```python
from build123d import *

# Parameters (mm, degrees)
BOSS_EXTRUDE1_START     = -1.5
BOSS_EXTRUDE1_DEPTH     = 1.8
SKETCH8_R               = 3
SKETCH8_R_2             = 2.5
BOSS_EXTRUDE2_DEPTH     = 1.2
CUT_EXTRUDE1_DEPTH      = 9.631338251
CUT_EXTRUDE1_DEPTH_BACK = 9.631338251
SKETCH9_R               = 2.5
FILLET1_R               = 0.254
SWEEP1_PITCH            = 0.8
SPLIT1_START            = -2.7460001
SPLIT1_OUTLINE_W        = 9
SPLIT1_OUTLINE_H        = 2.5
SPLIT1_DEPTH            = 5.4920002


with BuildPart() as part:
    # Sketch7 → Boss-Extrude1 (new body)
    with BuildSketch(Plane.XY.offset(BOSS_EXTRUDE1_START)):
        with BuildLine():
            Line((-6.42820323, 4), (6.42820323, 4))
            ThreePointArc((6.42820323, 4), (7.5, 0), (6.42820323, -4))
            Line((6.42820323, -4), (-6.42820323, -4))
            ThreePointArc((-6.42820323, -4), (-7.5, 0), (-6.42820323, 4))
        make_face()
    extrude(amount=BOSS_EXTRUDE1_DEPTH)

    # Sketch8 → Boss-Extrude2 (add)
    with BuildSketch(Plane.XY.offset(0.3)):
        with Locations((1.5, 0)):
            Circle(SKETCH8_R)
        with Locations((1.5, 0)):
            Circle(SKETCH8_R_2, mode=Mode.SUBTRACT)
    extrude(amount=BOSS_EXTRUDE2_DEPTH)

    # Sketch9 → Cut-Extrude1 (cut, two sides: drawn at the far end of the back side and taken through both)
    with BuildSketch(Plane.XY.offset(-CUT_EXTRUDE1_DEPTH_BACK)):
        with Locations((1.5, 0)):
            Circle(SKETCH9_R)
    extrude(amount=CUT_EXTRUDE1_DEPTH + CUT_EXTRUDE1_DEPTH_BACK, mode=Mode.SUBTRACT)

    # Fillet1
    fillet1_edges = [part.edges().sort_by_distance(p)[0] for p in [
        (-1.5, 0, 1.5),
    ]]
    fillet(fillet1_edges, radius=FILLET1_R)

    # Sweep1: arcs per turn and ends read off the stored shape
    # Sweep1: the profile of Sketch3 screwed along a right-hand helix through 4.75 turns, 8 arcs to a turn; built about Z, then put on its axis
    sweep1_z = Axis((0, 0, 0), (0, 0, 1))
    sweep1_corners = [(2.54330127, 0, 0.025), (2.54330127, 0, -0.725), (1.980384758, 0, -0.4), (1.980384758, 0, -0.3)]
    with BuildLine(mode=Mode.PRIVATE) as sweep1_profile:
        Line(sweep1_corners[0], sweep1_corners[1])
        Line(sweep1_corners[1], sweep1_corners[2])
        Line(sweep1_corners[2], sweep1_corners[3])
        Line(sweep1_corners[3], sweep1_corners[0])
    sweep1_cap = Face(sweep1_profile.wire())
    sweep1_turn_angles = [0, 22.5, 45, 67.5, 90, 112.5, 135, 157.5, 180, 202.5, 225, 247.5, 270, 292.5, 315, 337.5, 360]
    sweep1_turn_weights = [1, 0.9238795325112867, 1, 0.9238795325112867, 1, 0.9238795325112867, 1, 0.9238795325112867, 1, 0.9238795325112867, 1, 0.9238795325112867, 1, 0.9238795325112867, 1, 0.9238795325112867, 1]
    sweep1_turn_rails = [Edge.make_bspline([Vector(p[0], p[1], 0).rotate(sweep1_z, sweep1_turn_angles[k]) / sweep1_turn_weights[k] + Vector(0, 0, p[2] + SWEEP1_PITCH * sweep1_turn_angles[k] / 360) for k in range(17)], [0, 0, 0, 1, 1, 2, 2, 3, 3, 4, 4, 5, 5, 6, 6, 7, 7, 8, 8, 8], 2, sweep1_turn_weights) for p in sweep1_corners]
    sweep1_turn_sides = [Face.make_surface_from_curves(sweep1_turn_rails[p[0]], sweep1_turn_rails[p[1]]) for p in [(0, 1), (1, 2), (2, 3), (3, 0)]]
    sweep1_last_angles = [1440, 1462.5, 1485, 1507.5, 1530, 1552.5, 1575, 1597.5, 1620, 1642.5, 1665, 1687.5, 1710]
    sweep1_last_weights = [1, 0.9238795325112867, 1, 0.9238795325112867, 1, 0.9238795325112867, 1, 0.9238795325112867, 1, 0.9238795325112867, 1, 0.9238795325112776, 1]
    sweep1_last_rails = [Edge.make_bspline([Vector(p[0], p[1], 0).rotate(sweep1_z, sweep1_last_angles[k]) / sweep1_last_weights[k] + Vector(0, 0, p[2] + SWEEP1_PITCH * sweep1_last_angles[k] / 360) for k in range(13)], [0, 0, 0, 1, 1, 2, 2, 3, 3, 4, 4, 5, 5, 6, 6, 6], 2, sweep1_last_weights) for p in sweep1_corners]
    sweep1_last_sides = [Face.make_surface_from_curves(sweep1_last_rails[p[0]], sweep1_last_rails[p[1]]) for p in [(0, 1), (1, 2), (2, 3), (3, 0)]]
    sweep1 = Plane(origin=(1.5, 0, -1.5), x_dir=(0, 1, 0), z_dir=(0, 0, 1)) * Solid(Shell([*[p.moved(Location((0, 0, SWEEP1_PITCH * i))) for i in range(4) for p in sweep1_turn_sides], *sweep1_last_sides, sweep1_cap, sweep1_cap.rotate(sweep1_z, 1710).moved(Location((0, 0, SWEEP1_PITCH * 1710 / 360)))]))
    add(sweep1)

    # Split1: read off the stored shape, not the designer's step
    # Split1 outline → Split1 (cut)
    with BuildSketch(Plane(origin=(0, 0, 0), x_dir=(1, 0, 0), z_dir=(0, 1, 0)).offset(SPLIT1_START)):
        with Locations((1.5, -2.75)):
            Rectangle(SPLIT1_OUTLINE_W, SPLIT1_OUTLINE_H)
        with Locations((1.5, 2.75)):
            Rectangle(SPLIT1_OUTLINE_W, SPLIT1_OUTLINE_H)
    extrude(amount=SPLIT1_DEPTH, mode=Mode.SUBTRACT)

    # Cut-Extrude2 cone 1 section (through the dimple's axis) → Cut-Extrude2 (revolve, cut)
    with BuildSketch(Plane(origin=(1.5, 0, -1.5), x_dir=(0, 1, 0), z_dir=(1, 0, 0))):
        Polygon((0, 0), (2.5, 0), (0, 2.5), align=None)
    revolve(axis=Axis((1.5, 0, -1.5), (0, 0, 1)), mode=Mode.SUBTRACT)

    # Cut-Extrude3 cone 1 section (through the dimple's axis) → Cut-Extrude3 (revolve, cut)
    with BuildSketch(Plane(origin=(1.5, 0, 1.5), x_dir=(0, -1, 0), z_dir=(1, 0, 0))):
        Polygon((0, 0), (2.5, 0), (0, 2.5), align=None)
    revolve(axis=Axis((1.5, 0, 1.5), (0, 0, -1)), mode=Mode.SUBTRACT)


solid = part.part
```
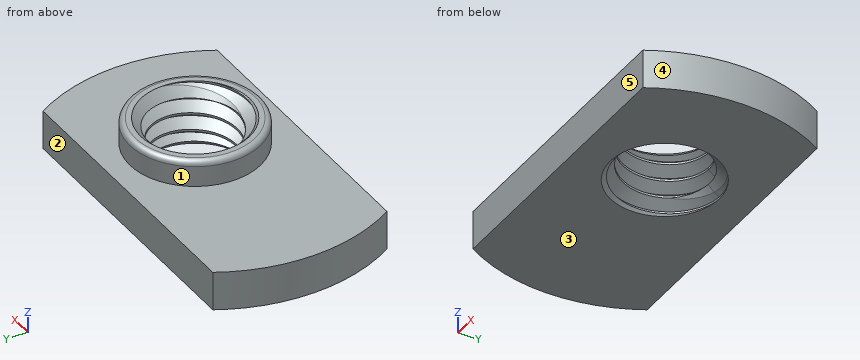
Geometry: final body of the model. Coordinates: model frame, mm. Face numbers are marked on the shaded views. A direction names the side the tool comes from. Round coordinates to 2 decimals unless told otherwise and drop trailing zeros. Write each loop counter-clockwise with the first axis right and the second up, starting at its lowest first coordinate (ties: lowest second). Pieces come first, ordered by that corner, then holes.
Item 1: Pin query (flat end, axial travel): P1, Ø1, axis at x = -2.5, z = 1, coming from the -Y side. Return the tip coordinate at first contact, or that it passes through.
Item 2: Section query B-B (x = -4.75). Return loops of the section in (y, z).
Item 3: Material intervals for L1, parallel to Z at x = -1.75, y = -3.25; L2, parallel to Y at x = 1.25, z = -1.2; L3, parallel to X at y = 0.5, z = 0.9, sorted ascending.
Item 4: Section query A-A (y = 3.25). Return loops of the section in (x, z), plus the area to 3 significant figures.
Item 5: Mould query, pull axis Y, two halves, no side actions, for the marked faces 3, 4 and 5. Classes: +Y half, -Y half, draft (parallel to the pull), parting line (faces both ways), or undercut.
Item 6: Set-up query: the marked faces 1 and 2. Return all of +Z, -Z, +X, -X, +Y, -Y with unobstructed straight access to the full face (end or side cutting, diameter ignored); none if empty.
Completed:
1. P1: passes through
2. outline: (-4, -1.5) - (4, -1.5) - (4, 0.3) - (-4, 0.3) - close
3. L1: z = -1.5 to 0.3
3. L2: y = -4 to -2.34, 2.19 to 4
3. L3: x = -1.46 to -0.65, 3.82 to 4.46
4. outline: (-6.81, -1.5) - (6.81, -1.5) - (6.81, 0.3) - (-6.81, 0.3) - close
4. area: 24.5 mm2
5. face 3: draft
5. face 4: parting line
5. face 5: -Y half
6. face 1: +Z
6. face 2: +Z, -Z, +X, -X, +Y
